Geometry check sheet. Reference: the model listing, model coordinates, mm. A direction names the side the tool comes from. Coordinates: 2 decimals unless noted, no trailing zeros. Order: outer loops, then holes, each group sorted by start corner. A loop starts at its lowest first (then second) coordinate and runs counter-clockwise, first axis right, second up. Notation, with made-up numbers: (25.5, 2.5) - (30.5, 2.5) arc R14 cw to (30.5, 21.5) - close; hole circle Ø4 at (36.25, 30.25). An arc over 180 degrees is marked (long way). Use CSV: the item, a comma, the result in double quotes. Start each with the question number.
1) Thickness scan on probe 1 along X at (y, z) = (68, -312); probe 2 along Y at (x, z) = (-5, -43); probe 3 along X at (y, z) = (68, -160). Record the ranges inside material, lowest first. Write a range as [from, to].
2) Sectioned sample at C-C, the plane z = -160. Record the cut outline in (x, y), and give its area (3 significant figures).
3) Sectioned sample at B-B, the plane y = 41. Record the cut outline in (x, z), and give its area (3 significant figures).
4) Draft check along Z on faces 1 (the flat face through (-101, 15, -15)), 2 (the cylindrical face through (-7.79, 68.52, -317.95)), 3 (the flat face through (-200, 35, -158)), 4 (the flat face through (-101, 8, -313)). Enter one of: released by +Z, released by -Z, zero draft, split by the parting line, or undercut.
5) Sectioned sample at D-D, the plane x = -54.5. Record the cut outline in (y, z).
6) Tool access check on faces 5 (the flat face through (-7, 63.533, -170)), 6 (the flat face through (-98.81, 13.76, -30.38)), 7 (the flat face through (-101.19, 28.992, -22.222)). Record the directions out of +Z, -Z, +X, -X, +Y, -Y that give a thin tool (end or side, any length) a straight path to the whole face; none if there is none.
7) Depth check by flat-ended pin: P1, Ø8, axis at x = -108, y = 11.5, coming from the +Z side; P2, Ø14, axis at x = -7.01, z = -8, coming from the -Y side; P3, Ø3, axis at x = -134.5, z = -114, coming from the +Y side; P4, Ø18.5, axis at y = 44, z = -109.5, coming from the +X side. Enter the tip coordinate at first touch or a pass-through.
8) Sectioned sample at A-A, the plane z = -128. Record the cut outline in (x, y).
Autodesk Inventor part; units mm, degrees
ref_plane "YZ Plane" through (0, 0, 0) normal (1, 0, 0) x (0, 1, 0)
ref_plane "XZ Plane" through (0, 0, 0) normal (0, 1, 0) x (-1, 0, 0)
ref_plane "XY Plane" through (0, 0, 0) normal (0, 0, 1) x (1, 0, 0)
sketch "Sketch1" plane through (0, 0, 0) normal (0, 1, 0) x (-1, 0, 0)
  line L0 (0, 0) -> (200, 0)
  line L1 (200, 0) -> (200, -320)
  line L2 (200, -320) -> (0, -320)
  line L3 (0, -320) -> (0, 0)
  dimension "d0" = 200
  dimension "d1" = 320
extrude "Extrusion1" add sketch "Sketch1" along normal blind 70
chamfer "Chamfer1" distance 30 angle 45 1 edges at (-100, 0, 0)
shell "Shell1" thickness 15 removed faces 1 at (-66.6667, 70, -106.6667)
sketch "Sketch5" plane through (0, 70, 0) normal (0, 1, 0) x (1, 0, 0)
  circle A0 centre (-192.9908, 160) radius 6
  line L0 (-200, 0) -> (0, 0)
  circle A1 centre (-192.9908, 8) radius 6
  circle A2 centre (-192.9908, 312) radius 6
  line L1 (-100, -14.4089) -> (-100, 373.6947) construction
  circle A3 centre (-7.0092, 160) radius 6
  circle A4 centre (-7.0092, 8) radius 6
  circle A5 centre (-7.0092, 312) radius 6
  dimension "d40" = 12
  dimension "d41" = 160
  dimension "d42" = 12
  dimension "d43" = 152
  dimension "d44" = 12
  dimension "d45" = 152
extrude "Extrusion5" cut sketch "Sketch5" against normal blind 3
chamfer "Chamfer2" distance 15 angle 45 1 edges at (-100, 0, -320)
sketch "Sketch6" plane through (0, 70, 0) normal (1, 0, 0) x (0, 0, -1)
  circle A0 centre (43, -45) radius 12.5
  line L0 (0, 0) -> (320, 0)
  line L1 (0, -40) -> (0, 0)
  line L2 (320, 0) -> (0, 0)
  line L3 (160, 0) -> (160, -70) construction
  circle A1 centre (277, -45) radius 12.5
  point P0 (0, -70)
  dimension "d51" = 25
  dimension "d52" = 45
  dimension "d53" = 43
sketch "Sketch8" plane through (-185, 15, -36.2132) normal (0, 1, 0) x (1, 0, 0)
  line L0 (170, 0) -> (170, 268.7868)
  line L1 (0, 0) -> (170, 0)
  line L2 (170, 0) -> (170, 268.7868)
  line L3 (170, 268.7868) -> (0, 268.7868)
  line L4 (0, 268.7868) -> (0, 0)
  point P0 (185, -36.2132)
extrude "Extrusion6" cut sketch "Sketch8" against normal blind 5
sketch "Sketch9" plane through (-15, 36.2132, -15) normal (0, 0.7071068, -0.7071068) x (-1, 0, 0)
  line L0 (-0.7971, -12.8149) -> (-1.097, -36.2132)
  line L1 (185, -36.2132) -> (-15, -36.2132)
  line L2 (0, -33.5355) -> (170, -33.5355)
  line L3 (170, 23.8909) -> (170, -181.1701)
  line L4 (0, -33.5355) -> (170, -33.5355)
  line L5 (170, -33.5355) -> (170, -20.1439)
  line L6 (170, -20.1439) -> (0, -20.1439)
  line L7 (0, -20.1439) -> (0, -33.5355)
  point P0 (-15, -15)
extrude "Extrusion7" cut sketch "Sketch9" against normal blind 5
extrude "Extrusion8" cut sketch "Sketch6" against normal blind 220
sketch "Sketch10" plane through (0, 70, -320) normal (0, 0, -1) x (-1, 0, 0)
  point P0 (0, -70)
sketch "Sketch11" plane through (0, 70, -320) normal (0, 0, -1) x (-1, 0, 0)
  point P0 (0, -70)
sketch "Sketch12" plane through (0, 70, 0) normal (0, 1, 0) x (1, 0, 0)
  point P0 (0, 0)
sketch "Sketch13" plane through (0, 70, 0) normal (1, 0, 0) x (0, 0, -1)
  point P0 (0, -70)
sketch "Sketch14" plane through (0, 70, -320) normal (0, 0, -1) x (-1, 0, 0)
  point P0 (0, -70)
sketch "Sketch15" plane through (0, 70, 0) normal (1, 0, 0) x (0, 0, -1)
  point P0 (0, -70)
sketch "Sketch16" plane through (0, 70, 0) normal (1, 0, 0) x (0, 0, -1)
  line L0 (41.7462, -8.2025) -> (302.1648, -8.2025) construction
  line L1 (41.7462, -6.4667) -> (302.1648, -6.4667)
  line L2 (302.1648, -9.9384) -> (41.7462, -9.9384)
  arc A0 (41.7462, -6.4667) -> (41.7462, -9.9384) centre (41.7462, -8.2025) ccw
  arc A1 (302.1648, -9.9384) -> (302.1648, -6.4667) centre (302.1648, -8.2025) ccw
  point P0 (0, -70)
  point P1 (171.9555, -8.2025)
extrude "Extrusion10" cut sketch "Sketch16" against normal blind 20
sketch "Sketch18" plane through (-200, 70, -320) normal (-1, 0, 0) x (0, 0, 1)
  line L0 (15, -60) -> (15, 0)
  line L1 (277.9177, -6.1098) -> (17, -6.1098)
  line L2 (15, -8.1098) -> (15, -7.8958)
  line L3 (17, -9.8958) -> (277.9177, -9.8958)
  line L4 (279.9177, -7.8958) -> (279.9177, -8.1098)
  arc A0 (17, -6.1098) -> (15, -8.1098) centre (17, -8.1098) ccw
  arc A1 (15, -7.8958) -> (17, -9.8958) centre (17, -7.8958) ccw
  arc A2 (279.9177, -8.1098) -> (277.9177, -6.1098) centre (277.9177, -8.1098) ccw
  arc A3 (277.9177, -9.8958) -> (279.9177, -7.8958) centre (277.9177, -7.8958) ccw
  point P0 (320, -70)
  point P1 (15, -9.8958)
  point P2 (15.0029, -8.0028)
  point P3 (279.9148, -8.0028)
  dimension "d65" = 2
extrude "Extrusion11" cut sketch "Sketch18" against normal blind 20 contours A0 L1 A2 A3 L3 A1
properties material "ABS Plastic"
Evaluation:
1,probe 1,"[-200, -198.99], [-186.99, -13.01], [-1.01, 0]"
1,probe 2,"[0, 12.5], [37.5, 60.06], [63.53, 70]"
1,probe 3,"[-200, -198.99], [-186.99, -185], [-15, -13.01], [-1.01, 0]"
2,outline,"(-200, 0) - (0, 0) - (0, 60.06) - (-15, 60.06) - (-15, 10) - (-185, 10) - (-185, 60.1) - (-200, 60.1) - close; (-200, 63.89) - (-185, 63.89) - (-185, 70) - (-186.99, 70) - (-186.99, 67) - (-198.99, 67) - (-198.99, 70) - (-200, 70) - close; (-15, 63.53) - (0, 63.53) - (0, 70) - (-1.01, 70) - (-1.01, 67) - (-13.01, 67) - (-13.01, 70) - (-15, 70) - close"
2,area,"3,620 mm²"
3,outline,"(-200, -320) - (0, -320) - (0, 0) - (-200, 0) - close; hole (-185, -305) - (-15, -305) - (-15, -15) - (-185, -15) - close"
3,area,"14,700 mm²"
4,face 1,"released by +Z"
4,face 2,"undercut"
4,face 3,"zero draft"
4,face 4,"released by -Z"
5,outline,"(0, -305) - (15, -320) - (70, -320) - (70, -305) - (10, -305) - (10, -36.21) - (8.96, -35.18) - (18.43, -25.71) - (21.97, -29.24) - (36.21, -15) - (70, -15) - (70, 0) - (30, 0) - (0, -30) - close"
6,face 5,"+X, -X"
6,face 6,"none"
6,face 7,"+Y"
7,P1,"z = -14.5"
7,P2,"y = 15"
7,P3,"y = 10"
7,P4,"x = 0"
8,outline,"(-200, 0) - (0, 0) - (0, 60.06) - (-15, 60.06) - (-15, 10) - (-185, 10) - (-185, 60.1) - (-200, 60.1) - close; (-200, 63.89) - (-185, 63.89) - (-185, 70) - (-200, 70) - close; (-15, 63.53) - (0, 63.53) - (0, 70) - (-15, 70) - close"
